Geometry check sheet. Reference: the model listing, model coordinates, mm. Face numbers are marked on the shaded views. A direction names the side the tool comes from. Round coordinates to 2 decimals unless told otherwise and drop trailing zeros. Order: outer loops, then holes, each group sorted by start corner. A loop starts at its lowest first (then second) coordinate and runs counter-clockwise, first axis right, second up. Notation, with made-up numbers: (13, 30) - (55, 30) arc R27 cw to (55, 55) - close; hole circle Ø3 at (-31, -15.5). An arc over 180 degrees is marked (long way). Return JSON: item names as keys, results as strings. Group by question number.
Q1. Sectioned sample at C-C, the plane y = -11. Give the number of separate pieces and of enclosed holes in the cut face, then the cut area to 3 significant figures.
Q2. Sectioned sample at D-D, the plane z = 24. Record the cut outline in (x, y) (3 decimals).
Q3. Tool access check on the marked faces 5 and 6. Record the directions out of +Z, -Z, +X, -X, +Y, -Y that give a thin tool (end or side, any length) a straight path to the whole face; none if there is none.
Q4. Sectioned sample at A-A, the plane z = 10.16. Record the cut outline in (x, y) (1 decimal), then the cut area to 3 significant figures.
Q5. Sectioned sample at B-B, the plane x = 19. Record the cut outline in (y, z).
Q6. Draft check along Z on the marked faces 1, 2, 3 and 4. Enter one of: pulls with the +Z half, pulls with the -Z half, needs draft (parallel to the pull), parting line crosses it, or undercut.
Q7. Material ranges on line 1 along Z through (x, y) = (47, -11); line 2 along X through (y, z) = (-0.5, 16.5) (3 decimals); line 3 along Z through (x, y) = (59, -4.5), recorded low to high.
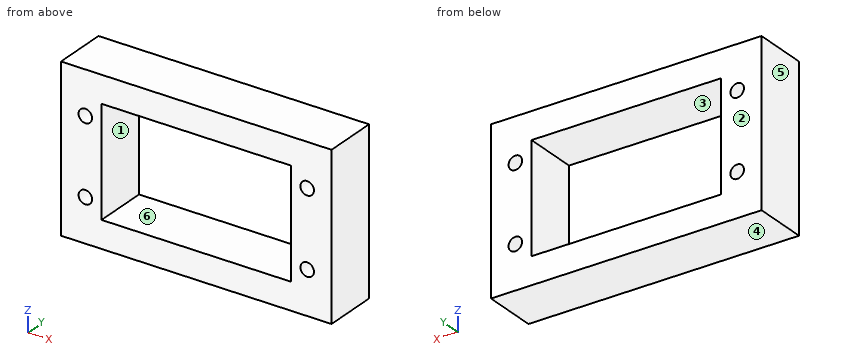
```python
from build123d import *

# Parameters (mm, degrees)
F0_W     = 63.5
F0_H     = 38.1
F0_R     = 1.5875
F0_W_2   = 44.45
F0_H_2   = 25.4
F1_DEPTH = 12.7


with BuildPart() as f1:
    # F0 (on Front) → F1 (new body)
    with BuildSketch(Plane.XZ):
        with Locations((31.75, 19.05)):
            Rectangle(F0_W, F0_H)
        with Locations((5.715, 10.16)):
            Circle(F0_R, mode=Mode.SUBTRACT)
        with Locations((57.785, 10.16)):
            Circle(F0_R, mode=Mode.SUBTRACT)
        with Locations((5.715, 27.94)):
            Circle(F0_R, mode=Mode.SUBTRACT)
        with Locations((31.75, 19.05)):
            Rectangle(F0_W_2, F0_H_2, mode=Mode.SUBTRACT)
        with Locations((57.785, 27.94)):
            Circle(F0_R, mode=Mode.SUBTRACT)
    extrude(amount=F1_DEPTH)


solid = f1.part
```
Reply:
{
 "1": {"separate pieces": "1", "enclosed holes": "5", "area": "1,260 mm^2"},
 "2": {"outline": "(0, -12.7) - (9.525, -12.7) - (9.525, 0) - (0, 0) - close; (53.975, -12.7) - (63.5, -12.7) - (63.5, 0) - (53.975, 0) - close"},
 "3": {"face 5": "+Z, -Z, -X, +Y, -Y", "face 6": "+Y, -Y"},
 "4": {"outline": "(0, -12.7) - (4.1, -12.7) - (4.1, 0) - (0, 0) - close; (7.3, -12.7) - (9.5, -12.7) - (9.5, 0) - (7.3, 0) - close; (54, -12.7) - (56.2, -12.7) - (56.2, 0) - (54, 0) - close; (59.4, -12.7) - (63.5, -12.7) - (63.5, 0) - (59.4, 0) - close", "area": "161 mm^2"},
 "5": {"outline": "(-12.7, 0) - (0, 0) - (0, 6.35) - (-12.7, 6.35) - close; (-12.7, 31.75) - (0, 31.75) - (0, 38.1) - (-12.7, 38.1) - close"},
 "6": {"face 1": "undercut", "face 2": "needs draft", "face 3": "undercut", "face 4": "pulls with the -Z half"},
 "7": {"line 1": "0 to 6.35, 31.75 to 38.1", "line 2": "0 to 9.525, 53.975 to 63.5", "line 3": "0 to 9.14, 11.18 to 26.92, 28.96 to 38.1"}
}
